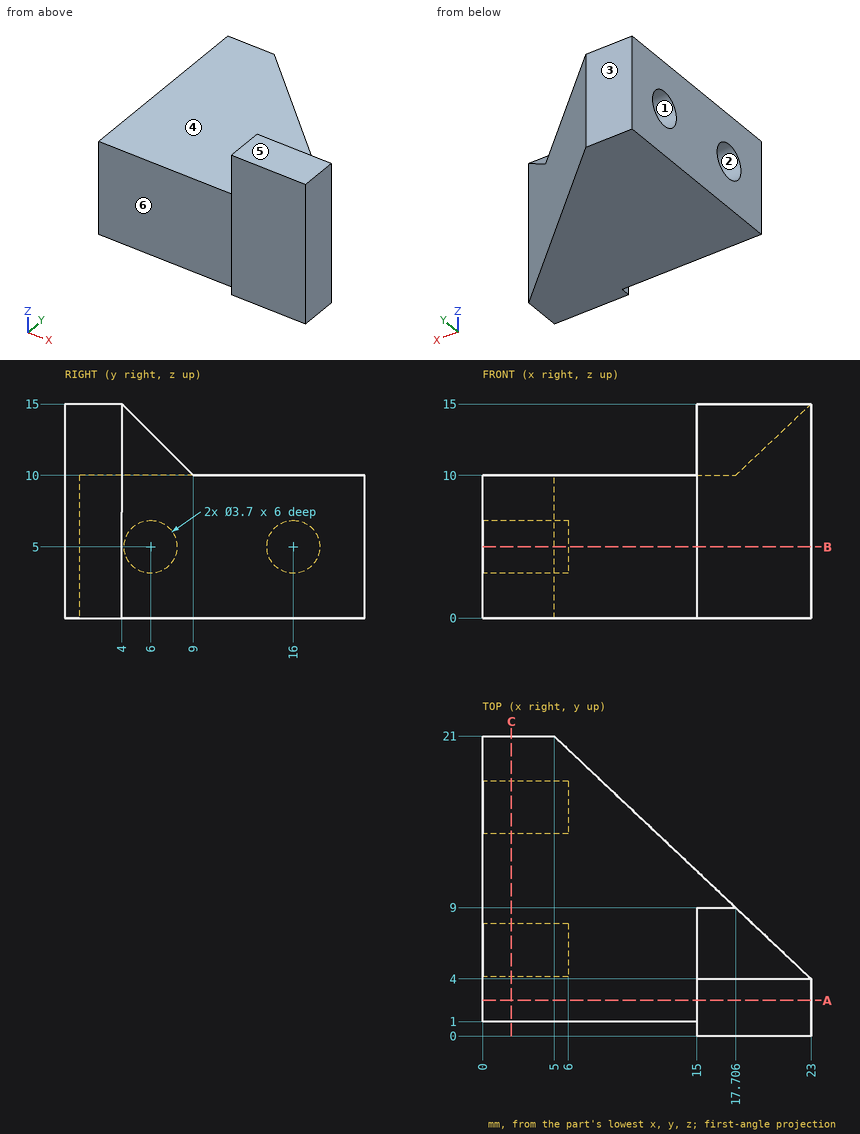
Answer from the drawing. Dimensions are ordinates in mm from the lowest x, y and z of the part. A direction names the side the tool comes from. Coordinates: 2 decimals unless noted, no trailing zeros. Order: outer loops, then holes, each group sorted by start corner. A loop starts at its lowest first (then second) coordinate and runs counter-clockwise, first axis right, second up. Notation, with made-up numbers: (-18, 49.5) - (28, 49.5) arc R14 cw to (28, 69.5) - close; hole circle Ø5 at (80.25, -18.75). An arc over 180 degrees is marked (long way). Answer as a JSON object with one key per item and string values. Group by question number.
Item 1: The mould has two halves that part along Y. Classify the marked faces 1, 2, 3 and 4: +Y half, -Y half, draft (parallel to the pull), parting line (faces both ways), or undercut.
Item 2: Section A-A (y = 2.5) is taken. Give the vertices of the cut face in (x, z).
Item 3: Consider probe 1 along Y at (x, z) = (3.45, 5); probe 2 along Z at (x, y) = (6.75, 11.25); probe 3 along Y at (x, z) = (3.5, 2). Determine where each line is inside the solid, lowest interval first. Write a range as from..to.
Item 4: Flat-ended cylindrical pins translate along their axes: P1, Ø2.5, axis at y = 5.5, z = 5, coming from the -X side; P2, Ø8, axis at x = 9, z = 5, coming from the -Y side; P3, Ø6, axis at y = 7.5, z = 11, coming from the +X side. Find the tip coordinate at first contact, or state that the pin passes through.
Item 5: A tool of negligible diameter and unlimited length cuts with its end or side. For the marked faces 5 and 6, from which of +Z, -Z, +X, -X, +Y, -Y can it reach the whole face along a straight path? Write none if from no direction.
Item 6: Section C-C (x = 2) is taken. Give the vertices of the cut face in (y, z).
Item 7: Section B-B (z = 5) is taken. Give the vertices of the cut face in (x, y).
Results are:
{
 "1": {"face 1": "undercut", "face 2": "undercut", "face 3": "+Y half", "face 4": "draft"},
 "2": {"outline": "(0, 0) - (23, 0) - (23, 15) - (15, 15) - (15, 10) - (0, 10) - close"},
 "3": {"probe 1": "y = 1..4.15, 7.85..14.15, 17.85..21", "probe 2": "z = 0..10", "probe 3": "y = 1..21"},
 "4": {"P1": "stops at x = 6", "P2": "stops at y = 1", "P3": "stops at x = 22.47"},
 "5": {"face 5": "+Z, +X, -X, +Y, -Y", "face 6": "+Z, -Z, -X, -Y"},
 "6": {"outline": "(1, 0) - (21, 0) - (21, 10) - (1, 10) - close; hole circle Ø3.7 at (6, 5); hole circle Ø3.7 at (16, 5)"},
 "7": {"outline": "(0, 1) - (15, 1) - (15, 0) - (23, 0) - (23, 4) - (5, 21) - (0, 21) - (0, 17.85) - (6, 17.85) - (6, 14.15) - (0, 14.15) - (0, 7.85) - (6, 7.85) - (6, 4.15) - (0, 4.15) - close"}
}
